Here's how the part is built. I have some questions about the finished solid (model axes, mm). A direction names the side the tool comes from. Coordinates: 2 decimals unless noted, no trailing zeros. Write each loop counter-clockwise with the first axis right and the second up, starting at its lowest first coordinate (ties: lowest second). Pieces come first, ordered by that corner, then holes. Notation, with made-up numbers: (76, 0.5) -> (87, 0.5) arc R14 ccw to (87, 18.5) -> close; hole circle Ø6 at (18.5, 7.5). An arc over 180 degrees is marked (long way). Use a Markdown table: item, result. Add a question column.
Item 1: On a 3-axis mill with a long thin cutter (end or side, diameter ignored), from which of +Z, -Z, +X, -X, +Y, -Y can I reach the whole of each face in a straight line? I mean faces 1 (the flat face through (-31, 190, -3.175)), 2 (the flat face through (-130.39, 139.85, 2.35)). Say none if no direction works.
Item 2: Imagine slicing it at A-A, the plane z = -1.5. Write out the boundary of the cut face in (x, y).
Item 3: Imagine slicing it at C-C, the plane y = 188. Write out the boundary of the cut face in (x, z) (1 decimal).
Item 4: Imagine slicing it at B-B, the plane y = 153.5. Write out the boundary of the cut face in (x, z), and give its area (3 significant figures).
Item 5: If I drill on line 1 along X through (y, z) = (195.5, -1.75); line 2 along Y through (x, z) = (73, 4.25); line 3 along Y through (x, z) = (28.5, -2.25), over which ranges is the centre line in solid material (lowest first)? Write a range as from..to.
Item 6: Imagine slicing it at D-D, the plane x = -21. Write out the boundary of the cut face in (y, z).
Item 7: Will these pins go through, and if not, where does the flat tip stop? pin 1 Ø1.4 at (x, z) = (-11.5, 1.5) entering from -Y; pin 2 Ø1 at (y, z) = (189, -2) entering from +X; pin 3 Ø3.5 at (y, z) = (189, -2) entering from -X.
Item 8: If we mould it in two halves opening along X, with no side actions, what happens to faces 3 (the flat face through (129.794, 140.882, 2.348)), 4 (the flat face through (32, 190, -3.175)), 5 (the flat face through (-134.57, 180.87, 2.35))? For each: pulls with the +X half, pulls with the -X half, needs draft (parallel to the pull), parting line crosses it, or undercut.
```python
from build123d import *

# Parameters (mm, degrees)
BOSS_EXTRUDE1_DEPTH = 4.7625
CUT_EXTRUDE2_DEPTH  = 271.489940724
SKETCH3_W           = 12.192
SKETCH3_H           = 15.24
BOSS_EXTRUDE2_DEPTH = 3.175


with BuildPart() as part:
    # Sketch1 → Boss-Extrude1 (new body)
    with BuildSketch(Plane.XY):
        Polygon((-122.047, 202.560020285), (-179.197, 103.573316632), (-151.334076009, 103.573316632), (-108.848772846, 177.160020285), (108.848772846, 177.160020285), (151.334076009, 103.573316632), (179.197, 103.573316632), (122.047, 202.560020285), (41.573947838, 202.560020285), (41.591522776, 199.385068928), (-41.591522776, 199.385068928), (-41.573947838, 202.560020285), align=None)
    extrude(amount=BOSS_EXTRUDE1_DEPTH)

    # Sketch2 → Cut-Extrude2 (cut, through all)
    with BuildSketch(Plane.XY.offset(4.7625)):
        Polygon((183.007, 96.974203056), (181.632184671, 96.180453056), (146.072184671, 157.772179773), (147.447, 158.565929773), align=None)
        Polygon((-183.007, 96.974203056), (-181.632184671, 96.180453056), (-146.072184671, 157.772179773), (-147.447, 158.565929773), align=None)
    extrude(amount=-CUT_EXTRUDE2_DEPTH, mode=Mode.SUBTRACT)

    # Sketch3 → Boss-Extrude2 (add)
    with BuildSketch(Plane(origin=(0, 0, 0), x_dir=(-1, 0, 0), z_dir=(0, 0, -1))):
        with Locations((-31.496, 189.733068928)):
            Rectangle(SKETCH3_W, SKETCH3_H)
        with Locations((31.496, 189.733068928)):
            Rectangle(SKETCH3_W, SKETCH3_H)
    extrude(amount=BOSS_EXTRUDE2_DEPTH)


solid = part.part
```
Ans:
| question | item | result |
|---|---|---|
| 1 | face 1 | -Z, +X, -X, +Y, -Y |
| 1 | face 2 | +Z, -Z, -Y |
| 2 | outline | (-37.59, 182.11) -> (-25.4, 182.11) -> (-25.4, 197.35) -> (-37.59, 197.35) -> close; (25.4, 182.11) -> (37.59, 182.11) -> (37.59, 197.35) -> (25.4, 197.35) -> close |
| 3 | outline | (-130.5, 0) -> (-37.6, 0) -> (-37.6, -3.2) -> (-25.4, -3.2) -> (-25.4, 0) -> (25.4, 0) -> (25.4, -3.2) -> (37.6, -3.2) -> (37.6, 0) -> (130.5, 0) -> (130.5, 4.8) -> (-130.5, 4.8) -> close |
| 4 | outline | (-148.54, 0) -> (-122.51, 0) -> (-122.51, 4.76) -> (-148.54, 4.76) -> close; (122.51, 0) -> (148.54, 0) -> (148.54, 4.76) -> (122.51, 4.76) -> close |
| 4 | area | 248 mm^2 |
| 5 | line 1 | x = -37.59..-25.4, 25.4..37.59 |
| 5 | line 2 | y = 177.16..202.56 |
| 5 | line 3 | y = 182.11..197.35 |
| 6 | outline | (177.16, 0) -> (199.39, 0) -> (199.39, 4.76) -> (177.16, 4.76) -> close |
| 7 | pin 1 | stops at y = 177.16 |
| 7 | pin 2 | stops at x = 37.59 |
| 7 | pin 3 | stops at x = -37.59 |
| 8 | face 3 | undercut |
| 8 | face 4 | needs draft |
| 8 | face 5 | pulls with the -X half |
